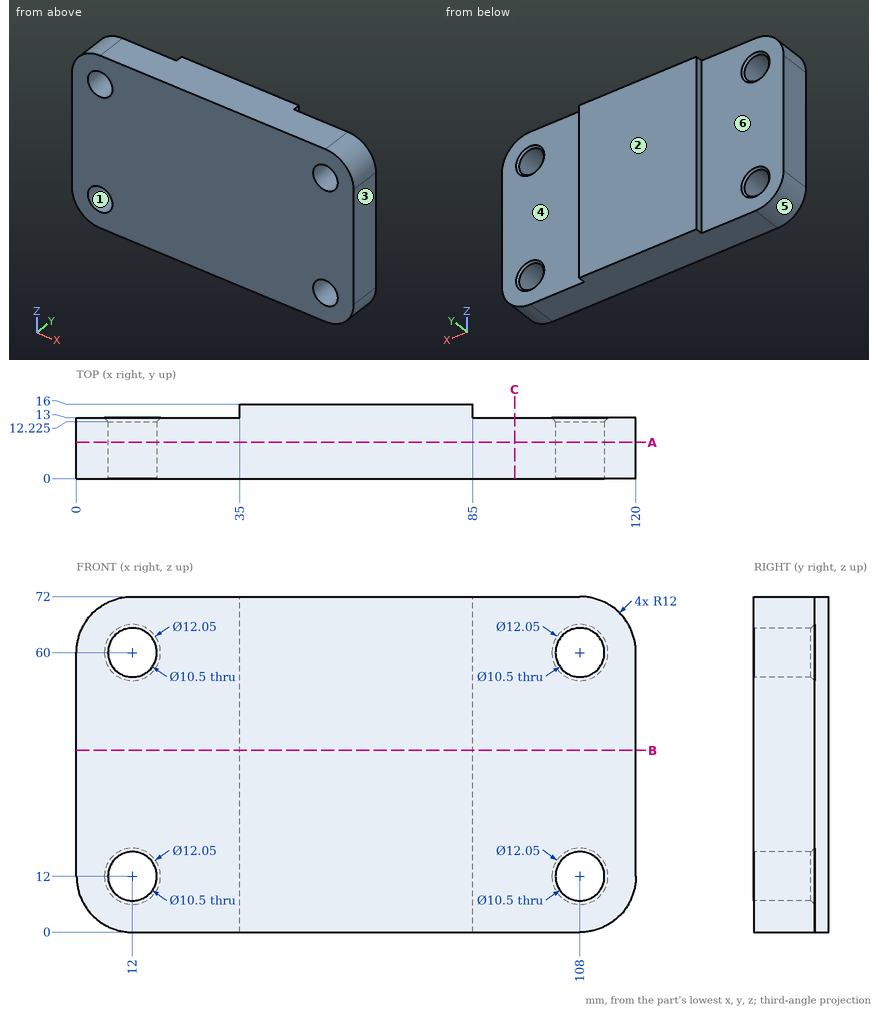
Job drawing, mm, ordinate dimensions from the low corner. One solid piece. A direction names the side the tool comes from. Round coordinates to 2 decimals unless told otherwise and drop trailing zeros. Order: outer loops, then holes, each group sorted by start corner. A loop starts at its lowest first (then second) coordinate and runs counter-clockwise, first axis right, second up. Notation, with made-up numbers: (-8.75, 68) -> (35.25, 68) arc R33 cw to (35.25, 98) -> close; hole circle Ø2 at (65, 56). An arc over 180 degrees is marked (long way). Answer in a Markdown table with one row per item.
1) Wall check: L1, parallel to Z at x = 108, y = 4.5; L2, parallel to X at y = 5.75, z = 60; L3, parallel to X at y = 2.5, z = 10.5. Give the ranges that are in metal, low to high.
Values:
| item | result |
|---|---|
| L1 | 0 to 6.75, 17.25 to 54.75, 65.25 to 72 |
| L2 | 0 to 6.75, 17.25 to 102.75, 113.25 to 120 |
| L3 | 0.09 to 6.97, 17.03 to 102.97, 113.03 to 119.91 |
2) Which spindle directions (+Z, -Z, +X, -X, +Y, -Y) get a long thin tool onto all of the face, cutting with end or side? Do the marked faces 4, 5 and 6. Say none if no direction does.
Values:
| item | result |
|---|---|
| face 4 | +Z, -Z, +X, +Y |
| face 5 | -Z, -X, +Y, -Y |
| face 6 | +Z, -Z, -X, +Y |
3) Band-saw the part on C-C on x = 94. Give the cut face in (y, z).
Values:
| item | result |
|---|---|
| outline | (0, 0) -> (13, 0) -> (13, 72) -> (0, 72) -> close |
4) Pin check, flat tips, straight feed: P1, Ø0.9, axis at y = 14.5, z = 52.5, coming from the -X side; P2, Ø0.9, axis at y = 14, z = 40, coming from the +X side; P3, Ø9.5, axis at x = 108, z = 12, coming from the +Y side; P4, Ø10.5, axis at x = 95.5, z = 38, coming from the +Y side. Stop position of each tip, or through.
Values:
| item | result |
|---|---|
| P1 | x = 35 |
| P2 | x = 85 |
| P3 | through |
| P4 | y = 13 |
5) Band-saw the part on B-B on z = 39. Give the cut face in (x, y).
Values:
| item | result |
|---|---|
| outline | (0, 0) -> (120, 0) -> (120, 13) -> (85, 13) -> (85, 16) -> (35, 16) -> (35, 13) -> (0, 13) -> close |
6) Band-saw the part on A-A on y = 7.75. Give the cut face in (x, z).
Values:
| item | result |
|---|---|
| outline | (0, 12) arc R12 ccw to (12, 0) -> (108, 0) arc R12 ccw to (120, 12) -> (120, 60) arc R12 ccw to (108, 72) -> (12, 72) arc R12 ccw to (0, 60) -> close; hole circle Ø10.5 at (12, 12); hole circle Ø10.5 at (12, 60); hole circle Ø10.5 at (108, 12); hole circle Ø10.5 at (108, 60) |
7) Mould opens along X. For the marked faces 1, 2 and 3 say: released by +X, released by -X, zero draft, split by the parting line, or undercut.
Values:
| item | result |
|---|---|
| face 1 | undercut |
| face 2 | zero draft |
| face 3 | released by +X |
